from build123d import *

# Parameters (mm, degrees)
F5_W     = 150
F5_H     = 6
F6_DEPTH = 1820
F8_D     = 23


with BuildPart() as f2:
    # F2: sweep along a path in F1
    with BuildLine(Plane.XY) as f2_path:
        Line((0, 0), (0, 1100))
        Line((0, 1100), (1860, 1100))
        Line((1860, 1100), (1860, 0))
    # F0 (on Front) → F2 (sweep)
    with BuildSketch(Plane.XZ):
        with BuildLine():
            Line((-15, -20), (15, -20))
            ThreePointArc((15, -20), (18.5355339059, -18.5355339059), (20, -15))
            Line((20, -15), (20, 15))
            ThreePointArc((20, 15), (18.5355339059, 18.5355339059), (15, 20))
            Line((15, 20), (-15, 20))
            ThreePointArc((-15, 20), (-18.5355339059, 18.5355339059), (-20, 15))
            Line((-20, 15), (-20, -15))
            ThreePointArc((-20, -15), (-18.5355339059, -18.5355339059), (-15, -20))
        make_face()
        with BuildLine():
            ThreePointArc((-15, -17.5), (-16.767766953, -16.767766953), (-17.5, -15))
            Line((-17.5, -15), (-17.5, 15))
            ThreePointArc((-17.5, 15), (-16.767766953, 16.767766953), (-15, 17.5))
            Line((-15, 17.5), (15, 17.5))
            ThreePointArc((15, 17.5), (16.767766953, 16.767766953), (17.5, 15))
            Line((17.5, 15), (17.5, -15))
            ThreePointArc((17.5, -15), (16.767766953, -16.767766953), (15, -17.5))
            Line((15, -17.5), (-15, -17.5))
        make_face(mode=Mode.SUBTRACT)
    sweep(path=f2_path.line, transition=Transition.RIGHT)

    # F3 (on face) → F4 (join, up to the next surface of F2)
    with BuildSketch(Plane.YZ.offset(20)):
        with BuildLine():
            Line((485, -20), (515, -20))
            ThreePointArc((515, -20), (518.5355339059, -18.5355339059), (520, -15))
            Line((520, -15), (520, 15))
            ThreePointArc((520, 15), (518.5355339059, 18.5355339059), (515, 20))
            Line((515, 20), (485, 20))
            ThreePointArc((485, 20), (481.4644660941, 18.5355339059), (480, 15))
            Line((480, 15), (480, -15))
            ThreePointArc((480, -15), (481.4644660941, -18.5355339059), (485, -20))
        make_face()
        with BuildLine():
            ThreePointArc((485, -17.5), (483.232233047, -16.767766953), (482.5, -15))
            Line((482.5, -15), (482.5, 15))
            ThreePointArc((482.5, 15), (483.232233047, 16.767766953), (485, 17.5))
            Line((485, 17.5), (515, 17.5))
            ThreePointArc((515, 17.5), (516.767766953, 16.767766953), (517.5, 15))
            Line((517.5, 15), (517.5, -15))
            ThreePointArc((517.5, -15), (516.767766953, -16.767766953), (515, -17.5))
            Line((515, -17.5), (485, -17.5))
        make_face(mode=Mode.SUBTRACT)
    extrude(until=Until.NEXT)

    # F5 (on face) → F6 (join, through all)
    with BuildSketch(Plane.YZ.offset(20)):
        with Locations((115, 0.7091578767)):
            Rectangle(F5_W, F5_H)
    extrude(amount=F6_DEPTH)

    # F8 (through all)
    with Locations(Plane(origin=(0, 1120, 0), x_dir=(-1, 0, 0), z_dir=(0, 1, 0))):
        with Locations((0, 0), (-1860, 0)):
            Hole(F8_D / 2)


solid = f2.part
Part model, mm, in its own coordinate system. A direction names the side the tool comes from. Give positions to 0.01 mm unless a question says otherwise; leave off trailing zeros.
1) Cut at A-A on y = 436.5. State how many separate pieces and enclosed holes the cut face has, then the cut area to 3 significant figures.
Resolved:
separate pieces: 2
enclosed holes: 2
area: 718 mm2
2) Which spindle directions (+Z, -Z, +X, -X, +Y, -Y) get a long thin tool onto all of the face, cutting with end or side? Do faces 3 (the face through (926, 1092, -20)), 4 (the face through (917, 114, -2.291)), 5 (the face through (934, 1097, -17.5)). Say none if no direction does.
Resolved:
face 3: -Z, +X, -X, +Y, -Y
face 4: -Z, -Y
face 5: none
3) Probe L1, parallel to Y at x = 1343, z = -12; L2, parallel to X at y = 717, z = -10.5; L3, parallel to Z at x = 0, y = 1119.2. List the from-to ranges inside material, lowest first.
Resolved:
L1: y = 480 to 482.5, 517.5 to 520, 1080 to 1082.5, 1117.5 to 1120
L2: x = -20 to -17.5, 17.5 to 20, 1840 to 1842.5, 1877.5 to 1880
L3: z = -17.71 to -11.5, 11.5 to 17.71
4) Pin check, flat tips, straight feed: pin 1 (1.5 mm diameter, centred on x = 478, z = -13, fed in from -Y); pin 2 (2.5 mm diameter, centred on y = 492, z = 17.5, fed in from -X). Stop position of each tip, or through.
Resolved:
pin 1: stops at y = 480
pin 2: stops at x = -19.84
5) Two-plate mould, pull along X, no slides. Class faces 1 (the face through (-18, 0, 0)), 2 (the face through (917, 114, 3.709)): released by +X, released by -X, zero draft, split by the parting line, or undercut.
Resolved:
face 1: zero draft
face 2: undercut
